For this review, use the dimensioned drawing (mm, ordinates from the lowest corner) and the shaded views. Coordinates: 2 decimals unless noted, no trailing zeros. Order: outer loops, then holes, each group sorted by start corner. A loop starts at its lowest first (then second) coordinate and runs counter-clockwise, first axis right, second up. Notation, with made-up numbers: (42, -34) -> (87, -34) arc R21 cw to (87, -18) -> close; hole circle Ø9 at (-18, 64). An arc over 180 degrees is marked (long way). Use one line per item in the form item = value. Start each with the question number.
(1) Take a section at D-D (x = 71.5). State how many separate pieces and enclosed holes the cut face has, then the cut area to 3 significant figures.
(2) Take a section at C-C (x = 108). State the section outline as (y, z) points, then the cut area to 3 significant figures.
(3) Take a section at A-A (z = 72.5). State the section outline as (x, y) points, then the cut area to 3 significant figures.
(4) Mouldability with a two-part tool opening along X and no side actions: class the marked faces 1 and 2 as +X half, -X half, draft (parallel to the pull), parting line (faces both ways), or undercut.
(5) Wall thickness on line 1 along X through (y, z) = (41.5, 55.5); line 2 along Z through (x, y) = (76, 34); line 3 along X through (y, z) = (26, 105.5): over which ranges is each line inside the solid? List them lowest first.
(6) Take a section at B-B (y = 29.5). State the section outline as (x, z) points.
(7) Insertion check: pin 1 Ø2.5 at (y, z) = (41, 73.5) entering from +X; pin 2 Ø2 at (y, z) = (24, 103) entering from -X; pin 3 Ø4 at (y, z) = (40, 65.5) entering from -X. Each pin has a flat end and moves straight along its axis. Give the tip position at first contact, or say it passes through.
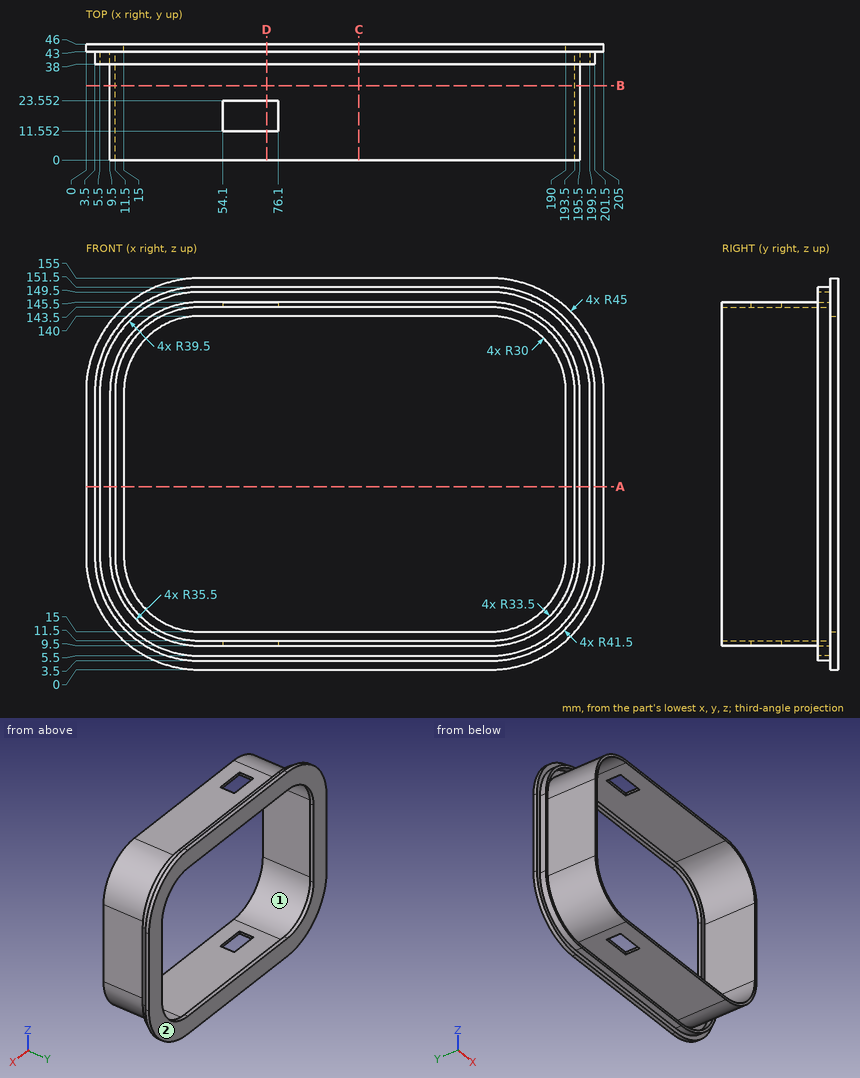
Findings:
q1.separate_pieces = 4
q1.enclosed_holes = 0
q1.area = 234 mm²
q2.outline = (0, 9.5) -> (43, 9.5) -> (43, 5.5) -> (38, 5.5) -> (38, 3.5) -> (43, 3.5) -> (43, 0) -> (46, 0) -> (46, 15) -> (43, 15) -> (43, 11.5) -> (0, 11.5) -> close; (0, 143.5) -> (43, 143.5) -> (43, 140) -> (46, 140) -> (46, 155) -> (43, 155) -> (43, 151.5) -> (38, 151.5) -> (38, 149.5) -> (43, 149.5) -> (43, 145.5) -> (0, 145.5) -> close
q2.area = 282 mm²
q3.outline = (0, 43) -> (3.5, 43) -> (3.5, 38) -> (5.5, 38) -> (5.5, 43) -> (9.5, 43) -> (9.5, 0) -> (11.5, 0) -> (11.5, 43) -> (15, 43) -> (15, 46) -> (0, 46) -> close; (190, 43) -> (193.5, 43) -> (193.5, 0) -> (195.5, 0) -> (195.5, 43) -> (199.5, 43) -> (199.5, 38) -> (201.5, 38) -> (201.5, 43) -> (205, 43) -> (205, 46) -> (190, 46) -> close
q3.area = 282 mm²
q4.face_1 = undercut
q4.face_2 = draft
q5.line_1 = 3.5 to 5.5, 9.5 to 11.5, 193.5 to 195.5, 199.5 to 201.5
q5.line_2 = 9.5 to 11.5, 143.5 to 145.5
q5.line_3 = 9.5 to 11.5, 193.5 to 195.5
q6.outline = (9.5, 45) arc R35.5 ccw to (45, 9.5) -> (160, 9.5) arc R35.5 ccw to (195.5, 45) -> (195.5, 110) arc R35.5 ccw to (160, 145.5) -> (45, 145.5) arc R35.5 ccw to (9.5, 110) -> close; hole (11.5, 45) arc R33.5 ccw to (45, 11.5) -> (160, 11.5) arc R33.5 ccw to (193.5, 45) -> (193.5, 110) arc R33.5 ccw to (160, 143.5) -> (45, 143.5) arc R33.5 ccw to (11.5, 110) -> close
q7.pin_1 = 201.5
q7.pin_2 = 9.5
q7.pin_3 = 3.5
